```python
from build123d import *

# Parameters (mm, degrees)
SKIZZE1_W                       = 42
SKIZZE1_H                       = 28
SKIZZE1_R                       = 3.5
AUFSATZ_LINEAR_AUSTRAGEN1_DEPTH = 8
SKIZZE2_R                       = 1.6
SCHNITT_LINEAR_AUSTRAGEN1_DEPTH = 15
M4_GEWINDEBOHRUNG1_D            = 3.3
M4_GEWINDEBOHRUNG1_DEPTH        = 15
M4_GEWINDEBOHRUNG1_TIP          = 0.991420021


with BuildPart() as part:
    # Skizze1 → Aufsatz-Linear austragen1 (new body)
    with BuildSketch(Plane.XY):
        with Locations((0.646863863, -0.143442623)):
            Rectangle(SKIZZE1_W, SKIZZE1_H)
        with Locations((0.646863863, -0.143442623)):
            Circle(SKIZZE1_R, mode=Mode.SUBTRACT)
    extrude(amount=AUFSATZ_LINEAR_AUSTRAGEN1_DEPTH)

    # Skizze2 → Schnitt-Linear austragen1 (cut)
    with BuildSketch(Plane.ZY.offset(20.353136137)):
        with Locations(Location((4, 5.856557377, 0), (0, 0, 270))):
            Circle(SKIZZE2_R)
        with Locations(Location((4, -6.143442623, 0), (0, 0, 270))):
            Circle(SKIZZE2_R)
    extrude(amount=-SCHNITT_LINEAR_AUSTRAGEN1_DEPTH, mode=Mode.SUBTRACT)

    # M4 Gewindebohrung1
    with Locations(Plane(origin=(-20.353136137, -6.143442623, 4), x_dir=(0, -1, 0), z_dir=(-1, 0, 0))):
        with Locations((0, 0), (-12, 0)):
            Hole(M4_GEWINDEBOHRUNG1_D / 2, depth=M4_GEWINDEBOHRUNG1_DEPTH)
            with Locations((0, 0, -(M4_GEWINDEBOHRUNG1_DEPTH + M4_GEWINDEBOHRUNG1_TIP / 2))):  # 118° drill point
                Cone(0, M4_GEWINDEBOHRUNG1_D / 2, M4_GEWINDEBOHRUNG1_TIP, mode=Mode.SUBTRACT)


solid = part.part
```
Verification items for the finished model (mm, model axes). A direction names the side the tool comes from. Coordinates: 2 decimals unless noted, no trailing zeros. Loops run counter-clockwise (first coordinate to the right, second up) from the corner with the lowest first, then second, coordinate; pieces in that order, holes last. Notation, with made-up numbers: (-20.75, 39) -> (-3.75, 39) arc R35 cw to (-3.75, 74) -> close; hole circle Ø10 at (-13.75, -32.5). An arc over 180 degrees is marked (long way). Put each result on its own line as item: value.
1. Thickness scan on line 1 (Y direction, x = -9.25, z = 4); line 2 (Y direction, x = -16, z = 3); line 3 (X direction, y = -2.5, z = 3). Record the ranges inside material, lowest first.
Result set:
line 1: y = -14.14 to -7.79, -4.49 to 4.21, 7.51 to 13.86
line 2: y = -14.14 to -7.46, -4.83 to 4.54, 7.17 to 13.86
line 3: x = -20.35 to -1.94, 3.23 to 21.65
2. Gauge pin test, flat end, axial feed: P1, Ø2, axis at y = 5.86, z = 4, coming from the -X side. Record the tip position at first contact, or that the pin passes through.
Result set:
P1: stops at x = -4.96
3. Section check A-A, the plane y = 1.75. Record the boundary of the cut face in (x, z), then the cut area to 3 significant figures.
Result set:
outline: (-20.35, 0) -> (-2.3, 0) -> (-2.3, 8) -> (-20.35, 8) -> close; (3.59, 0) -> (21.65, 0) -> (21.65, 8) -> (3.59, 8) -> close
area: 289 mm^2
4. Tool access check on faces 1 (the face through (5, 0, 8)), 2 (the face through (-12.75, 4.21, 4.07)). Record the directions out of +Z, -Z, +X, -X, +Y, -Y that give a thin tool (end or side, any length) a straight path to the whole face; none if there is none.
Result set:
face 1: +Z, +X, -X, +Y, -Y
face 2: -X
5. Section check C-C, the plane x = 0. Record the boundary of the cut face in (y, z), then the cut area to 3 significant figures.
Result set:
outline: (-14.14, 0) -> (-3.58, 0) -> (-3.58, 8) -> (-14.14, 8) -> close; (3.3, 0) -> (13.86, 0) -> (13.86, 8) -> (3.3, 8) -> close
area: 169 mm^2
6. Section check D-D, the plane z = 1. Record the boundary of the cut face in (x, y), then the cut area to 3 significant figures.
Result set:
outline: (-20.35, -14.14) -> (21.65, -14.14) -> (21.65, 13.86) -> (-20.35, 13.86) -> close; hole circle Ø7 at (0.65, -0.14)
area: 1,140 mm^2
7. Mould release check, pull along Y, two halves, no side actions. Record for faces 3 (the face through (0, 13.857, 4)), 4 (the face through (-12.75, -7.79, 4.07)), 5 (the face through (0, -14.143, 4)), 6 (the face through (-20.353, 0, 4)): pulls with the +Y half, pulls with the -Y half, needs draft (parallel to the pull), parting line crosses it, or undercut.
Result set:
face 3: pulls with the +Y half
face 4: undercut
face 5: pulls with the -Y half
face 6: needs draft
8. Section check B-B, the plane x = -17. Record the boundary of the cut face in (y, z).
Result set:
outline: (-14.14, 0) -> (13.86, 0) -> (13.86, 8) -> (-14.14, 8) -> close; hole circle Ø3.3 at (-6.14, 4); hole circle Ø3.3 at (5.86, 4)
